from build123d import *

# Parameters (mm, degrees)
F0_R     = 50.8
F0_R_2   = 12.7
F0_W     = 12.4153457582
F0_H     = 7.0944800973
F0_W_2   = 12.021208182
F0_H_2   = 7.4886232615
F1_DEPTH = 6.35


# Not quite as in the source:
# - a length typed as a fraction of an inch, garbled in the dataset ("3 / 203.2 mm" for 3/8 in), is restored


with BuildPart() as f1:
    # F0 (on Top) → F1 (new body, symmetric)
    with BuildSketch(Plane.XY):
        Circle(F0_R)
        Circle(F0_R_2, mode=Mode.SUBTRACT)
        with Locations((16.4552591741, -33.107586205)):
            Rectangle(F0_W, F0_H, mode=Mode.SUBTRACT)
        with Locations((-22.3673274741, 27.3925866932)):
            Rectangle(F0_W_2, F0_H_2, mode=Mode.SUBTRACT)
    extrude(amount=F1_DEPTH, both=True)


solid = f1.part
Geometry check sheet. Reference: the model listing, model coordinates, mm. A direction names the side the tool comes from. Give positions to 0.01 mm unless a question says otherwise; leave off trailing zeros. Order: outer loops, then holes, each group sorted by start corner. A loop starts at its lowest first (then second) coordinate and runs counter-clockwise, first axis right, second up. Notation, with made-up numbers: M 42,51 L 60,51 A17 cw 60,55 Z; hole C -15,-5 d10. An arc over 180 degrees is marked long. Use a Markdown table: item, result.
Item 1: Section check C-C (z = 4.5). Record the cut outline in (x, y), and give its area (3 significant figures).
Answers follow:
| item | result |
|---|---|
| outline | C 0,0 d101.6; hole M -28.38,23.65 L -16.36,23.65 L -16.36,31.14 L -28.38,31.14 Z; hole C 0,0 d25.4; hole M 10.25,-36.65 L 22.66,-36.65 L 22.66,-29.56 L 10.25,-29.56 Z |
| area | 7,420 mm2 |
Item 2: Section check A-A (x = 0). Record the cut outline in (y, z).
Answers follow:
| item | result |
|---|---|
| outline | M -50.8,-6.35 L -12.7,-6.35 L -12.7,6.35 L -50.8,6.35 Z; M 12.7,-6.35 L 50.8,-6.35 L 50.8,6.35 L 12.7,6.35 Z |
Item 3: Depth check by flat-ended pin: P1, Ø5.5, axis at y = -33, z = 2.5, coming from the -X side; P2, Ø2, axis at y = -32.5, z = 2.5, coming from the +X side; P3, Ø1, axis at y = 26, z = -4.5, coming from the -X side. Enter the tip coordinate at first touch or a pass-through.
Answers follow:
| item | result |
|---|---|
| P1 | stops at x = -40.81 |
| P2 | stops at x = 39.85 |
| P3 | stops at x = -43.94 |
Item 4: Draft check along Y on faces 1 (the flat face through (16, -36.655, 0)), 2 (the flat face through (11, -11, -6.35)), 3 (the cylindrical face through (-11.012, -49.592, 0.089)). Enter one of: +Y half, -Y half, draft (parallel to the pull), parting line (faces both ways), or undercut.
Answers follow:
| item | result |
|---|---|
| face 1 | undercut |
| face 2 | draft |
| face 3 | parting line |
Item 5: Tool access check on faces 4 (the flat face through (-28.378, 27, 0)), 5 (the flat face through (11, -11, 6.35)). Record the directions out of +Z, -Z, +X, -X, +Y, -Y that give a thin tool (end or side, any length) a straight path to the whole face; none if there is none.
Answers follow:
| item | result |
|---|---|
| face 4 | +Z, -Z |
| face 5 | +Z, +X, -X, +Y, -Y |
Item 6: Section check D-D (y = -39.5). Record the cut outline in (x, z).
Answers follow:
| item | result |
|---|---|
| outline | M -31.94,-6.35 L 31.94,-6.35 L 31.94,6.35 L -31.94,6.35 Z |
Item 7: Material ranges on line 1 along Y through (x, z) = (0, -0.25); line 2 along Y through (x, z) = (11, -4.5); line 3 along X through (y, z) = (26, -4.5), recorded low to high.
Answers follow:
| item | result |
|---|---|
| line 1 | y = -50.8 to -12.7, 12.7 to 50.8 |
| line 2 | y = -49.59 to -36.65, -29.56 to -6.35, 6.35 to 49.59 |
| line 3 | x = -43.64 to -28.38, -16.36 to 43.64 |
